CAD build for the part. Positions are in the model's coordinates, mm. Face numbers are marked on the shaded views. A direction names the side the tool comes from. Round coordinates to 2 decimals unless told otherwise and drop trailing zeros. Loops run counter-clockwise (first coordinate to the right, second up) from the corner with the lowest first, then second, coordinate; pieces in that order, holes last.
Autodesk Inventor part; units mm, degrees
ref_plane "YZ Plane" through (0, 0, 0) normal (1, 0, 0) x (0, 1, 0)
ref_plane "XZ Plane" through (0, 0, 0) normal (0, 1, 0) x (-1, 0, 0)
ref_plane "XY Plane" through (0, 0, 0) normal (0, 0, 1) x (1, 0, 0)
sketch "Sketch1" plane through (0, 0, 0) normal (0, 1, 0) x (-1, 0, 0)
  circle A0 centre (24, -57.282) radius 1.6
  circle A1 centre (-24, -57.282) radius 1.6
  circle A2 centre (30.6147, -73.9084) radius 1.6
  circle A3 centre (-30.6218, -73.9117) radius 1.6
  circle A4 centre (28.2679, -64.7437) radius 1.6
  circle A5 centre (-28.2698, -64.7437) radius 1.6
  line L0 (48.2265, -83.602) -> (45.2265, -83.602)
  line L1 (45.2265, -83.602) -> (45.2265, -77.602)
  line L2 (45.2265, -77.602) -> (48.2265, -77.602)
  line L3 (48.2265, -77.602) -> (48.2265, -83.602)
  line L4 (-45.2265, -83.602) -> (-48.2265, -83.602)
  line L5 (-48.2265, -83.602) -> (-48.2265, -77.602)
  line L6 (-48.2265, -77.602) -> (-45.2265, -77.602)
  line L7 (-45.2265, -77.602) -> (-45.2265, -83.602)
  line L8 (48.3297, -88.9448) -> (2.1402, -66.9582)
  line L9 (-2.1585, -66.9585) -> (-48.3297, -88.9448)
  arc A6 (2.1402, -66.9582) -> (-2.1585, -66.9585) centre (-0.0088, -71.4728) ccw
  line L10 (30.6147, -73.9084) -> (28.0518, -79.2924)
  line L11 (28.0518, -79.2924) -> (-28.0596, -79.2924)
  line L12 (-30.6218, -73.9117) -> (-28.0596, -79.2924)
  line L13 (-28.0596, -79.2924) -> (-28.9194, -77.4867)
  line L14 (28.0518, -79.2924) -> (28.9114, -77.4867)
  line L15 (2.9996, -65.1524) -> (21.6357, -74.0234)
  line L16 (-3.0185, -65.1529) -> (-21.6377, -74.0192)
  arc A7 (2.9996, -65.1524) -> (-3.0185, -65.1529) centre (-0.009, -71.4729) ccw
  line L17 (26.297, -68.8841) -> (23.4415, -74.883)
  line L18 (24.3011, -73.0771) -> (25.5905, -70.3683)
  line L19 (7.0641, -61.5496) -> (5.1533, -60.64)
  line L20 (-26.2983, -68.8839) -> (-24.3033, -73.0733)
  line L21 (-23.4434, -74.879) -> (-25.5914, -70.3683)
  line L22 (-5.1635, -60.6408) -> (-7.0717, -61.5494)
  arc A8 (5.1533, -60.64) -> (-5.1635, -60.6408) centre (-0.0043, -71.4751) ccw
  arc A9 (28.2679, -67.7437) -> (28.2679, -61.7437) centre (28.2679, -64.7437) ccw
  line L23 (28.2679, -64.7437) -> (28.2679, -61.7437) construction
  line L24 (28.2679, -64.7437) -> (31.2679, -64.7437) construction
  line L25 (28.2679, -64.7437) -> (28.2679, -67.7437) construction
  line L26 (28.2679, -61.7437) -> (7.9237, -61.7437)
  line L27 (28.2679, -67.7437) -> (28.1029, -67.7437)
  arc A10 (-28.2698, -61.7437) -> (-28.2698, -67.7437) centre (-28.2698, -64.7437) ccw
  line L28 (-28.2698, -64.7437) -> (-28.2698, -61.7437) construction
  line L29 (-28.2698, -64.7437) -> (-25.2698, -64.7437) construction
  line L30 (-28.2698, -67.7437) -> (-28.104, -67.7437)
  line L31 (-28.2698, -61.7437) -> (-7.9316, -61.7437)
  arc A11 (21.6357, -74.0234) -> (24.3011, -73.0771) centre (22.4953, -72.2175) ccw
  arc A12 (-24.3033, -73.0733) -> (-21.6377, -74.0192) centre (-22.4976, -72.2134) ccw
  arc A13 (-7.9316, -61.7437) -> (-7.0717, -61.5494) centre (-7.9316, -59.7437) ccw
  arc A14 (7.0641, -61.5496) -> (7.9237, -61.7437) centre (7.9237, -59.7437) ccw
  arc A15 (28.1029, -67.7437) -> (26.297, -68.8841) centre (28.1029, -69.7437) ccw
  arc A16 (-26.2983, -68.8839) -> (-28.104, -67.7437) centre (-28.104, -69.7437) ccw
  line L32 (28.2679, -61.7437) -> (-28.2698, -61.7437)
  point P0 (0, 0)
  dimension "d0" = 3.2
  dimension "d1" = 6
  dimension "d2" = 6
  dimension "d3" = 5
  dimension "d4" = 2
  dimension "d5" = 7
  dimension "d6" = 5
  dimension "d7" = 12
  dimension "d8" = 3
  dimension "d9" = 90
  dimension "d10" = 180
  dimension "d11" = 3
  dimension "d12" = 90
  dimension "d13" = 2
  dimension "d14" = 2
extrude "Extrusion1" add sketch "Sketch1" along normal blind 2.5 contours A7 L16 A12 L20 A16 L30 A10 L31 L32 L26 A9 L27 A15 L17 A11 L15
sketch "Sketch2" plane through (0, 2.5, 0) normal (0, 1, 0) x (1, 0, 0)
  line L0 (-24.3011, 73.0771) -> (-26.297, 68.8841)
  line L1 (26.2983, 68.8839) -> (24.3033, 73.0733)
  arc A0 (-21.6357, 74.0234) -> (-24.3011, 73.0771) centre (-22.4953, 72.2175) ccw
  line L2 (-24.4649, 72.7332) -> (-24.3011, 73.0771)
  arc A1 (-24.4649, 72.7332) -> (-23.5723, 70.0943) centre (-22.659, 71.8736) ccw
  line L3 (24.4662, 72.7312) -> (24.3033, 73.0733)
  arc A2 (23.5739, 70.0921) -> (24.4662, 72.7312) centre (22.6605, 71.8713) ccw
  arc A3 (24.3033, 73.0733) -> (21.6377, 74.0192) centre (22.4976, 72.2134) ccw
  line L4 (21.6377, 74.0192) -> (3.0185, 65.1529)
  line L5 (-2.9996, 65.1524) -> (-21.6357, 74.0234)
  arc A4 (-2.9996, 65.1524) -> (3.0185, 65.1529) centre (0.009, 71.4729) ccw
  line L6 (-28.2679, 61.7437) -> (28.2698, 61.7437)
  line L7 (7.742, 61.9645) -> (23.5739, 70.0921)
  line L8 (-7.7335, 61.9644) -> (-23.5723, 70.0943)
  line L9 (-6.8202, 61.7437) -> (6.8286, 61.7437)
  arc A5 (6.8286, 61.7437) -> (7.742, 61.9645) centre (6.8286, 63.7437) ccw
  arc A6 (-7.7335, 61.9644) -> (-6.8202, 61.7437) centre (-6.8202, 63.7437) ccw
  point P0 (0, 0)
  point P1 (-5.1533, 60.64)
  point P2 (-25.2991, 70.9806)
  point P3 (25.3008, 70.9786)
  point P4 (7.312, 61.7437)
  point P5 (-7.3035, 61.7437)
  dimension "d17" = 2
  dimension "d18" = 2
  dimension "d23" = 2
extrude "Extrusion2" add sketch "Sketch2" along normal blind 25
sketch "Sketch3" plane through (0, 27.5, 0) normal (0, 1, 0) x (1, 0, 0)
  arc A0 (23.5739, 70.0921) -> (24.4662, 72.7312) centre (22.6605, 71.8713) ccw
  arc A1 (28.2698, 61.7437) -> (28.2698, 67.7437) centre (28.2698, 64.7437) ccw
  line L0 (28.2698, 67.7437) -> (28.104, 67.7437)
  arc A2 (26.2983, 68.8839) -> (28.104, 67.7437) centre (28.104, 69.7437) ccw
  line L1 (26.2983, 68.8839) -> (24.4662, 72.7312)
  circle A3 centre (28.2698, 64.7437) radius 1.6
  arc A4 (23.5739, 70.0921) -> (24.4662, 72.7312) centre (22.6605, 71.8713) ccw
  line L2 (24.4662, 72.7312) -> (24.3033, 73.0733)
  arc A5 (24.3033, 73.0733) -> (21.6377, 74.0192) centre (22.4976, 72.2134) ccw
  line L3 (21.6377, 74.0192) -> (3.0185, 65.1529)
  arc A6 (-2.9996, 65.1524) -> (3.0185, 65.1529) centre (0.009, 71.4729) ccw
  line L4 (-2.9996, 65.1524) -> (-21.6357, 74.0234)
  arc A7 (-21.6357, 74.0234) -> (-24.3011, 73.0771) centre (-22.4953, 72.2175) ccw
  line L5 (-24.3011, 73.0771) -> (-24.4649, 72.7332)
  arc A8 (-24.4649, 72.7332) -> (-23.5723, 70.0943) centre (-22.659, 71.8736) ccw
  arc A9 (-24.4649, 72.7332) -> (-23.5723, 70.0943) centre (-22.659, 71.8736) ccw
  line L6 (-24.4649, 72.7332) -> (-26.297, 68.8841)
  arc A10 (-28.1029, 67.7437) -> (-26.297, 68.8841) centre (-28.1029, 69.7437) ccw
  line L7 (-28.1029, 67.7437) -> (-28.2679, 67.7437)
  arc A11 (-28.2679, 67.7437) -> (-28.2679, 61.7437) centre (-28.2679, 64.7437) ccw
  circle A12 centre (-28.2679, 64.7437) radius 1.6
  arc A13 (-7.7335, 61.9644) -> (-6.8202, 61.7437) centre (-6.8202, 63.7437) ccw
  line L8 (-7.7335, 61.9644) -> (-23.5723, 70.0943)
  line L9 (-28.2679, 61.7437) -> (-6.8202, 61.7437)
  line L10 (-23.5723, 70.0943) -> (-7.7335, 61.9644)
  arc A14 (-7.7335, 61.9644) -> (-6.8202, 61.7437) centre (-6.8202, 63.7437) ccw
  line L11 (-6.8202, 61.7437) -> (6.8286, 61.7437)
  arc A15 (6.8286, 61.7437) -> (7.742, 61.9645) centre (6.8286, 63.7437) ccw
  line L12 (7.742, 61.9645) -> (23.5739, 70.0921)
  arc A16 (6.8286, 61.7437) -> (7.742, 61.9645) centre (6.8286, 63.7437) ccw
  line L13 (6.8286, 61.7437) -> (28.2698, 61.7437)
  line L14 (23.5739, 70.0921) -> (7.742, 61.9645)
  point P0 (0, 0)
extrude "Extrusion3" add sketch "Sketch3" along normal blind 2.5
properties part number "Front guard v2"
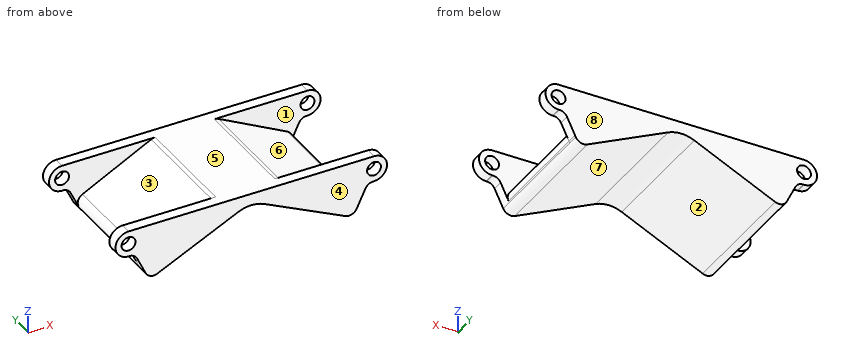
Item 1: Cut at C-C (x = -16). List the corners of the cut face in (y, z).
Verdict:
outline: (0, -71.34) - (30, -71.34) - (30, -61.74) - (27.5, -61.74) - (27.5, -66.21) - (2.5, -66.21) - (2.5, -61.74) - (0, -61.74) - close
Item 2: Wall check: L1, parallel to Y at x = -18, z = -63.5; L2, parallel to X at y = 20.5, z = -68.5; L3, parallel to X at y = 7, z = -65. Give the ranges that are in metal, low to high.
Verdict:
L1: y = 0 to 2.5, 27.5 to 30
L2: x = -20.47 to -10.03, 10.05 to 20.47
L3: x = -13.65 to -2.66, 2.67 to 13.65
Item 3: Flat gauge pins, fed straight in: P1, Ø2, axis at x = 10, y = 4.5, coming from the -Z side; P2, Ø2, axis at x = -20, y = 20, coming from the +Z side; P3, Ø2, axis at y = 24, z = -71, coming from the +X side. Where does each tip first touch, or does it go through?
Verdict:
P1: stops at z = -68.95
P2: stops at z = -67.75
P3: stops at x = 24.66
Item 4: Cut at A-A (y = 12.75). List the corners of the cut face in (x, z), plus the area to 3 significant figures.
Verdict:
outline: (-24.46, -72.73) - (-24.3, -73.08) arc R2 ccw to (-21.64, -74.02) - (-3, -65.15) arc R7 cw to (3.02, -65.15) - (21.64, -74.02) arc R2 ccw to (24.3, -73.07) - (24.47, -72.73) arc R2 ccw to (23.57, -70.09) - (7.74, -61.96) arc R2 ccw to (6.83, -61.74) - (-6.82, -61.74) arc R2 ccw to (-7.73, -61.96) - (-23.57, -70.09) arc R2 ccw to start
area: 228 mm2
Item 5: Mould opens along X. For the marked faces 6, 7 and 8 say: released by +X, released by -X, zero draft, split by the parting line, or undercut.
Verdict:
face 6: released by +X
face 7: undercut
face 8: zero draft
Item 6: Cut at B-B (z = -71.5). List the corners of the cut face in (x, y).
Verdict:
outline: (-25.05, 0) - (-16.33, 0) - (-16.33, 30) - (-25.05, 30) - (-25.05, 27.5) - (-24.62, 27.5) - (-24.62, 2.5) - (-25.05, 2.5) - close; (16.35, 0) - (25.05, 0) - (25.05, 2.5) - (24.63, 2.5) - (24.63, 27.5) - (25.05, 27.5) - (25.05, 30) - (16.35, 30) - close
Item 7: 3-axis set-ups, long thin cutter, end or side, ignore diameter. For the marked faces 1, 2, 3, 4 and 5: which of +Z, -Z, +X, -X, +Y, -Y reach the whole face in a straight line?
Verdict:
face 1: +Z, +X
face 2: -Z, +Y, -Y
face 3: +Z, -X
face 4: +Z, -Z, +X, -X, -Y
face 5: +Z, +X, -X, +Y, -Y
Item 8: Cut at D-D (x = 16). List the corners of the cut face in (y, z), plus the area to 3 significant figures.
Verdict:
outline: (0, -71.33) - (30, -71.33) - (30, -61.74) - (27.5, -61.74) - (27.5, -66.2) - (2.5, -66.2) - (2.5, -61.74) - (0, -61.74) - close
area: 176 mm2
